For this review, take the finished solid that the model builds, in its own axes (mm). A direction names the side the tool comes from. Give positions to 0.01 mm unless a question says otherwise; leave off trailing zeros. Loops run counter-clockwise (first coordinate to the right, second up) from the corner with the lowest first, then second, coordinate; pieces in that order, holes last. Notation, with made-up numbers: (55, 65) - (111, 65) arc R19 ccw to (111, 81) - close; hole circle Ø9 at (35, 74). An arc over 180 degrees is marked (long way). Answer in a Markdown table with one row per item.
```python
from build123d import *

# Parameters (mm, degrees)
SKETCH_2_R          = 3
SKETCH_2_R_2        = 1.5
SKETCH_2_R_3        = 2.5
EXTRUDE_1_DEPTH     = 3
EXTRUDE_2_DEPTH     = 196
SKETCH_5_R          = 8
CUT_EXTRUDE_1_DEPTH = 10
SKETCH_6_R          = 4.05
CUT_EXTRUDE_2_DEPTH = 10


with BuildPart() as part:
    # 草图2 → 凸台-拉伸1 (new body)
    with BuildSketch(Plane(origin=(0, 0, 0), x_dir=(0, 0, -1), z_dir=(1, 0, 0))):
        with BuildLine():
            Line((138.514809283, 84.200667909), (-11.70063651, 38.25042621))
            ThreePointArc((-11.70063651, 38.25042621), (-39.560188627, -5.915359313), (0, -40))
            Line((0, -40), (16.710190716, -40))
            Line((16.710190716, -40), (156.071648789, 40.329376559))
            Line((156.071648789, 40.329376559), (156.071648789, 43.792069046))
            ThreePointArc((156.071648789, 43.792069046), (165.334026038, 71.834783727), (138.514809283, 84.200667909))
        make_face()
        Circle(SKETCH_2_R, mode=Mode.SUBTRACT)
        with Locations((145, 70)):
            Circle(SKETCH_2_R_2, mode=Mode.SUBTRACT)
        with Locations((138, 63)):
            Circle(SKETCH_2_R_2, mode=Mode.SUBTRACT)
        with Locations((145, 56)):
            Circle(SKETCH_2_R_2, mode=Mode.SUBTRACT)
        with Locations((145, 63)):
            Circle(SKETCH_2_R_3, mode=Mode.SUBTRACT)
        with Locations((152, 63)):
            Circle(SKETCH_2_R_2, mode=Mode.SUBTRACT)
    extrude_1 = extrude(amount=EXTRUDE_1_DEPTH)

    # 草图4 → 凸台-拉伸2 (add)
    with BuildSketch(Plane(origin=(3, 0, 0), x_dir=(0, 0, -1), z_dir=(1, 0, 0))):
        with BuildLine():
            Line((0, -40), (16.710190716, -40))
            Line((16.710190716, -40), (156.071648789, 40.329376559))
            Line((156.071648789, 40.329376559), (156.071648789, 43.792069046))
            Line((156.071648789, 43.792069046), (19.975563357, -34.655113166))
            ThreePointArc((19.975563357, -34.655113166), (10.339136167, -38.640681455), (0, -40))
        make_face()
    extrude(amount=EXTRUDE_2_DEPTH)

    # 镜向2: 凸台-拉伸1 across plane
    add(extrude_1.mirror(Plane(origin=(101, 0, 0), x_dir=(0, 0, 1), z_dir=(1, 0, 0))))

    # 草图5 → 切除-拉伸1 (cut)
    with BuildSketch(Plane(origin=(202, 0, 0), x_dir=(0, 0, -1), z_dir=(1, 0, 0))):
        Circle(SKETCH_5_R)
    extrude(amount=-CUT_EXTRUDE_1_DEPTH, mode=Mode.SUBTRACT)

    # 草图6 → 切除-拉伸2 (cut)
    with BuildSketch(Plane.ZY):
        Circle(SKETCH_6_R)
    extrude(amount=-CUT_EXTRUDE_2_DEPTH, mode=Mode.SUBTRACT)


solid = part.part
```
1. We need section B-B, the plane z = -76. Give the boundary of the cut face in (x, y).
Values:
| item | result |
|---|---|
| outline | (0, -5.82) - (202, -5.82) - (202, 65.08) - (199, 65.08) - (199, -2.36) - (3, -2.36) - (3, 65.08) - (0, 65.08) - close |
2. Wall thickness on line 1 (Y direction, x = 201, z = -145); line 2 (X direction, y = 76, z = -132); line 3 (Y direction, x = 1, z = -138): over which ranges is each line inside the solid? List them lowest first. Write a range as [from, to].
Values:
| item | result |
|---|---|
| line 1 | y = [33.95, 54.5], [57.5, 60.5], [65.5, 68.5], [71.5, 85.17] |
| line 2 | x = [0, 3], [199, 202] |
| line 3 | y = [29.91, 61.5], [64.5, 84.04] |
3. Clearance check with flat-ended pins moving along their axes: pin 1 (1.8 mm diameter, centred on y = 70, z = -145, fed in from +X); pin 2 (8 mm diameter, centred on x = 111, z = -58, fed in from +Y); pin 3 (12 mm diameter, centred on x = 149, z = -96, fed in from +Y); pin 4 (5 mm diameter, centred on x = 115, y = 11.5, fed in from +Z). State where each tip first meets the part, or that it passes through.
Values:
| item | result |
|---|---|
| pin 1 | passes through |
| pin 2 | stops at y = -10.43 |
| pin 3 | stops at y = 12.62 |
| pin 4 | stops at z = -95.71 |
4. Mouldability with a two-part tool opening along Y and no side actions: class faces 4 (the face through (200.52, -5.13, 39.67)), 5 (the face through (200.521, 63.751, -147.385)), 6 (the face through (102, -40, -8)) as released by +Y, released by -Y, zero draft, split by the parting line, or undercut.
Values:
| item | result |
|---|---|
| face 4 | split by the parting line |
| face 5 | undercut |
| face 6 | released by -Y |
5. We need section D-D, the plane y = 74.5. Give the boundary of the cut face in (x, z), and give its area (3 significant figures).
Values:
| item | result |
|---|---|
| outline | (0, -163.95) - (3, -163.95) - (3, -106.8) - (0, -106.8) - close; (199, -163.95) - (202, -163.95) - (202, -106.8) - (199, -106.8) - close |
| area | 343 mm^2 |
6. For faces 1 (the face through (200.52, -7.81, 1.73)), 2 (the face through (99.63, 5.12, -88.98)), 3 (the face through (1.479, -3.954, -0.878)), list the 3-axis set-ups (+Z, -Z, +X, -X, +Y, -Y) from which the entire face can be reached by the end or side of a thin tool; tool diameter is ignored.
Values:
| item | result |
|---|---|
| face 1 | +X |
| face 2 | +Z, +Y |
| face 3 | +X, -X |
7. We need section C-C, the plane x = 132.5. Give the boundary of the cut face in (y, z), and give its area (3 significant figures).
Values:
| item | result |
|---|---|
| outline | (-40, -16.71) - (40.33, -156.07) - (43.79, -156.07) - (-34.66, -19.98) arc R40 cw to (-40, 0) - close |
| area | 503 mm^2 |
8. We need section A-A, the plane y = 0. Give the boundary of the cut face in (x, z).
Values:
| item | result |
|---|---|
| outline | (0, -86.11) - (202, -86.11) - (202, -8) - (199, -8) - (199, -80.1) - (3, -80.1) - (3, -4.05) - (0, -4.05) - close; (0, 4.05) - (3, 4.05) - (3, 40) - (0, 40) - close; (199, 8) - (202, 8) - (202, 40) - (199, 40) - close |
